Autodesk Inventor part; units mm, degrees
ref_plane "YZ Plane" through (0, 0, 0) normal (1, 0, 0) x (0, 1, 0)
ref_plane "XZ Plane" through (0, 0, 0) normal (0, 1, 0) x (-1, 0, 0)
ref_plane "XY Plane" through (0, 0, 0) normal (0, 0, 1) x (1, 0, 0)
sketch "スケッチ1" plane through (0, 0, 0) normal (0, 1, 0) x (-1, 0, 0)
  line L0 (25, 10) -> (-25, 10)
  line L1 (-25, 10) -> (-25, -10)
  line L2 (-25, -10) -> (25, -10)
  line L3 (25, -10) -> (25, 10)
  line L4 (25, 10) -> (-25, -10) construction
  line L5 (-25, 10) -> (25, -10) construction
  point P0 (0, 0)
  dimension "d0" = 20
  dimension "d1" = 50
extrude "押し出し1" add sketch "スケッチ1" along normal blind 5
sketch "スケッチ4" plane through (0, 5, 0) normal (0, 1, 0) x (1, 0, 0)
  line L0 (-25, -10) -> (25, -10)
  line L1 (-25, 10) -> (-25, -10)
  line L2 (25, -10) -> (25, 10)
  point P0 (0, 0)
  point P1 (-18, 0)
  dimension "d17" = 10
  dimension "d18" = 7
hole "穴2" at (-18, 5, 0) direction (0, -1, 0) diameter 6 end through all
sketch "スケッチ5" plane through (0, 5, 0) normal (0, 1, 0) x (1, 0, 0)
  line L0 (-10, 5) -> (25, 5)
  line L1 (25, 5) -> (25, -5)
  line L2 (25, -5) -> (-10, -5)
  line L3 (-10, -5) -> (-10, 5)
  line L4 (-25, 10) -> (-25, -10)
  point P0 (0, 0)
  dimension "d30" = 10
  dimension "d31" = 35
  dimension "d32" = 5
  dimension "d45" = 15
extrude "押し出し3" add sketch "スケッチ5" along normal blind 25
sketch "スケッチ6" plane through (0, 0, 0) normal (0, -1, 0) x (1, 0, 0)
  line L0 (-5, 2.75) -> (5, 2.75)
  line L1 (5, 2.75) -> (5, -2.75)
  line L2 (5, -2.75) -> (-5, -2.75)
  line L3 (-5, -2.75) -> (-5, 2.75)
  line L4 (-5, 2.75) -> (5, -2.75) construction
  line L5 (5, 2.75) -> (-5, -2.75) construction
  point P0 (0, 0)
  dimension "d35" = 10
  dimension "d36" = 5.5
extrude "押し出し4" add sketch "スケッチ6" along normal blind 3
sketch "スケッチ8" plane through (-10, 30, 5) normal (0, 0, 1) x (1, 0, 0)
  line L0 (10, -19) -> (35, -19)
  line L1 (35, -19) -> (35, -25)
  line L2 (35, -25) -> (10, -25)
  line L3 (10, -25) -> (10, -19)
  line L4 (30, -5) -> (30, -20)
  line L5 (35, -25) -> (35, 0)
  line L6 (-15, -25) -> (35, -25)
  point P0 (10, -30)
  dimension "d47" = 0
  dimension "d48" = 0
  dimension "d49" = 6
  dimension "d58" = 25
extrude "押し出し6" cut sketch "スケッチ8" against normal through all
sketch "スケッチ9" plane through (-10, 30, 5) normal (0, 0, 1) x (1, 0, 0)
  line L0 (30, -5) -> (10, -5)
  line L1 (10, -5) -> (10, -15)
  line L2 (10, -15) -> (30, -15)
  line L3 (30, -15) -> (30, -5)
  line L4 (0, 0) -> (35, 0)
  line L5 (35, -19) -> (35, 0)
  point P0 (10, -30)
  dimension "d52" = 5
  dimension "d53" = 5
  dimension "d54" = 20
  dimension "d55" = 10
extrude "押し出し7" cut sketch "スケッチ9" against normal through all
fillet "フィレット2" radius 2 38 edges at (-10, 17.5, 5) (10, 15, 5) (10, 15, -5) (12.5, 11, -5) (-10, 17.5, -5) (0, 11, 0) (0, 8, -5) (12.5, 11, 5) (0, 8, 5) (25, 20.5, 5) (25, 20.5, -5) (25, 11, 0) (20, 15, 0) (20, 20, 5) (20, 20, -5) (0, 15, 0) (-10, 30, 0) (0, 25, 0) (0, 20, -5) (7.5, 30, 5) (7.5, 30, -5) (10, 25, -5) (10, 25, 5) (0, 20, 5) (25, 30, 0) (20, 25, 0) (0, 5, 0) (-5, 5, 5) (-10, 5, 0) (-5, 5, -5) (0, 5, -10) (-25, 5, 0) (0, 5, 10) (-25, 2.5, -10) (-25, 2.5, 10) (25, 2.5, -10) (25, 5, 0) (25, 2.5, 10)
properties part number "cable_holder"
Model file for the job. Use its own axes, mm. A direction names the side the tool comes from. Coordinates: 2 decimals unless noted, no trailing zeros. Order: outer loops, then holes, each group sorted by start corner. A loop starts at its lowest first (then second) coordinate and runs counter-clockwise, first axis right, second up. Notation, with made-up numbers: (-26.75, 31.25) -> (19.25, 31.25) arc R20 ccw to (19.25, 41.25) -> close; hole circle Ø6 at (28, 33). An arc over 180 degrees is marked (long way). Return JSON: item names as keys, results as strings. Group by question number.
Item 1: Saw through at B-B on x = -18. Write the cut outline in (y, z), then the cut area to 3 significant figures.
Item 2: Saw through at C-C on y = 21. Write the cut outline in (x, z).
Item 3: Pull direction X, two halves, no side cores. Call faces 1 (the cylindrical face through (24.4, 20.61, 4.43)), 2 (the flat face through (0, 1, -10)), 3 (the cylindrical face through (9.89, 14.43, -4.4)): pulls with the +X half, pulls with the -X half, needs draft (parallel to the pull), parting line crosses it, or undercut.
Item 4: Saw through at A-A on z = 0. State how many separate pieces and enclosed holes the cut face has, then the cut area to 3 significant figures.
Item 5: Wall check: line 1 along X through (y, z) = (2.05, 0); line 2 along Y through (x, z) = (2.5, -3.5); line 3 along Z through (x, y) = (-18, 2.7). Give the ranges that are in metal, low to high. Write a range as [from, to].
Item 6: Flat gauge pins, fed straight in: P1, Ø10, axis at x = 9, y = 17.5, coming from the -Z side; P2, Ø2, axis at x = 7, z = 7, coming from the -Y side; P3, Ø9.5, axis at x = -18, z = 0, coming from the +Y side; P4, Ø1.5, axis at x = 15.5, y = 9.5, coming from the +Z side. Where does each tip first touch, or does it go through?
Item 7: Tool access for faces 4 (the cylindrical face through (20.57, 20.04, 4.4)), 5 (the cylindrical face through (0.57, 24.4, -0.04)), 6 (the flat face through (12, 11, 0)): list every direction of +Z, -Z, +X, -X, +Y, -Y with a clear straight run to the whole face (end or side of a thin tool).
Values found:
{
 "1": {"outline": "(0, -10) -> (3, -10) arc R2 ccw to (5, -8) -> (5, -3) -> (0, -3) -> close; (0, 3) -> (5, 3) -> (5, 8) arc R2 ccw to (3, 10) -> (0, 10) -> close", "area": "68.3 mm2"},
 "2": {"outline": "(-10, -3) arc R2 ccw to (-8, -5) -> (-2, -5) arc R2 ccw to (0, -3) -> (0, 3) arc R2 ccw to (-2, 5) -> (-8, 5) arc R2 ccw to (-10, 3) -> close; (20, -3) arc R2 ccw to (22, -5) -> (23, -5) arc R2 ccw to (25, -3) -> (25, 3) arc R2 ccw to (23, 5) -> (22, 5) arc R2 ccw to (20, 3) -> close"},
 "3": {"face 1": "pulls with the +X half", "face 2": "needs draft", "face 3": "undercut"},
 "4": {"separate pieces": "2", "enclosed holes": "1", "area": "777 mm2"},
 "5": {"line 1": "x = [-25, -21], [-15, 25]", "line 2": "y = [0, 5], [11.06, 14.94], [25.06, 29.94]", "line 3": "z = [-10, -3], [3, 10]"},
 "6": {"P1": "stops at z = -5", "P2": "stops at y = 0", "P3": "stops at y = 5", "P4": "passes through"},
 "7": {"face 4": "+Z", "face 5": "+Z, -Z", "face 6": "+Z, -Z, +X"}
}
